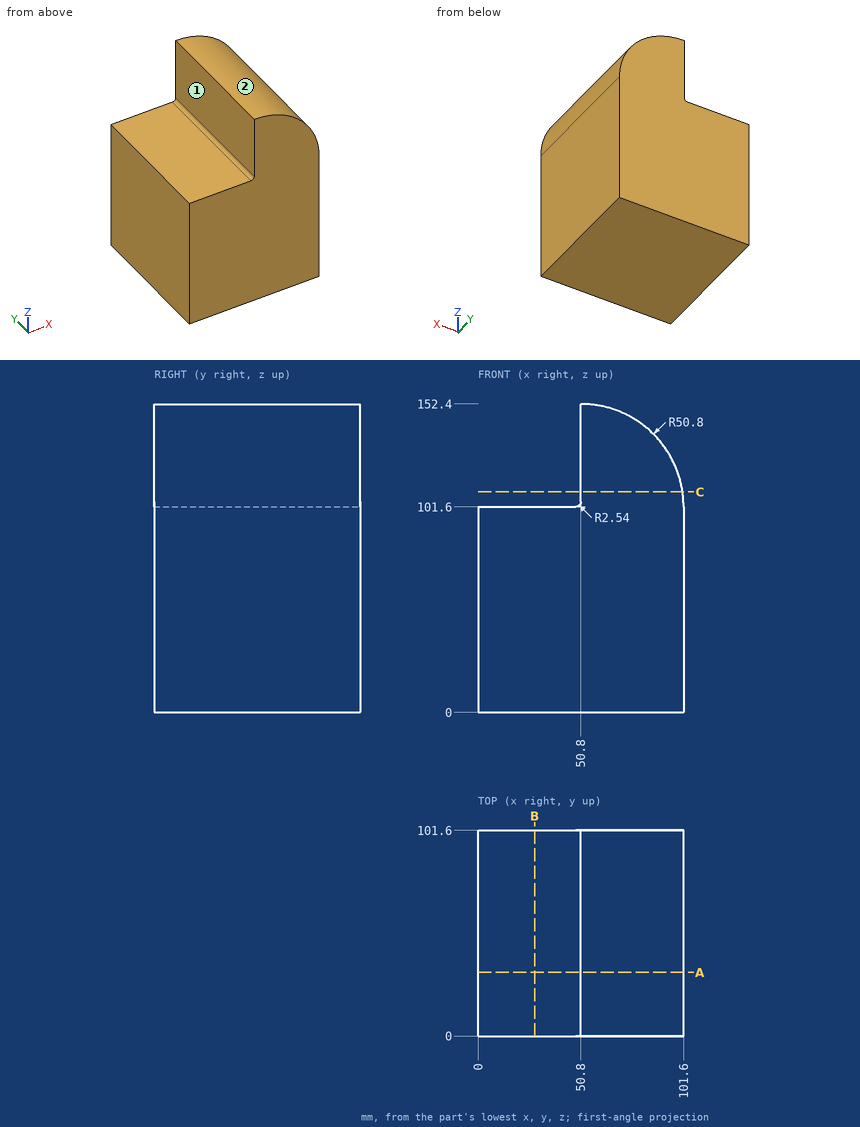
For this review, use the dimensioned drawing (mm, ordinates from the lowest corner) and the shaded views. A direction names the side the tool comes from. Give positions to 0.01 mm unless a question says otherwise; leave off trailing zeros. Order: outer loops, then holes, each group sorted by start corner. A loop starts at its lowest first (then second) coordinate and runs counter-clockwise, first axis right, second up. Notation, with made-up numbers: M 41.5,-16.75 L 48.5,-16.75 A23 cw 48.5,0.25 Z; hole C -4,43 d2. An arc over 180 degrees is marked long. One line per question, with ' | ' between items. Start each with the question number.
1) Clearance check with a flat-ended pin moving along its axis: P1, Ø10, axis at x = 20, y = 37, coming from the +Z side. State where the tip first meets the part, or that it passes through.
2) For the marked faces 1 and 2, list the 3-axis set-ups (+Z, -Z, +X, -X, +Y, -Y) from which the entire face can be reached by the end or side of a thin tool; tool diameter is ignored.
3) Consider section C-C, the plane z = 109. Give the boundary of the cut face in (x, y), then the cut area to 3 significant figures.
4) Wall thickness on L1, parallel to Z at x = 9.5, y = 52; L2, parallel to X at y = 12.5, z = 114.5; L3, parallel to Z at x = 94, y = 23.5: over which ranges is each line inside the solid? List them lowest first. Write a range as from..to.
5) Consider section A-A, the plane y = 31.5. Give the boundary of the cut face in (x, z), then the cut area to 3 significant figures.
6) Consider section B-B, the plane x = 28. Give the boundary of the cut face in (y, z).
Found:
1) P1: stops at z = 101.6
2) face 1: +Z, -X, +Y, -Y | face 2: +Z, +X, +Y, -Y
3) outline: M 50.8,0 L 101.06,0 L 101.06,101.6 L 50.8,101.6 Z | area: 5,110 mm²
4) L1: z = 0..101.6 | L2: x = 50.8..99.93 | L3: z = 0..128.33
5) outline: M 0,0 L 101.6,0 L 101.6,101.6 A50.8 ccw 50.8,152.4 L 50.8,104.14 A2.54 cw 48.26,101.6 L 0,101.6 Z | area: 12,400 mm²
6) outline: M 0,0 L 101.6,0 L 101.6,101.6 L 0,101.6 Z
